Work out the finished part from the listing and answer in its coordinate system (mm). A direction names the side the tool comes from. Round coordinates to 2 decimals unless told otherwise and drop trailing zeros. Write each loop counter-clockwise with the first axis right and the second up, starting at its lowest first coordinate (ties: lowest second). Pieces come first, ordered by that corner, then holes. Notation, with made-up numbers: M 74,-36.5 L 114,-36.5 A4 cw 114,-29.5 Z; hole C -1,62 d1. An arc over 180 degrees is marked long. One line per item, written item: value. Start each with the question number.
Q1. Find section C-C (y = 11). Write down the section's boundary in (x, z) (3 decimals), and give its area (3 significant figures).
Q2. The mould has two halves that part along Y. Classify faces 1 (the flat face through (-0.1, -2.5, 22.86)), 2 (the flat face through (0, -16, 16.51)), 3 (the cylindrical face through (24.85, 14.23, 19.64)): released by +Y, released by -Y, zero draft, split by the parting line, or undercut.
Q3. A tool of negligible diameter and unlimited length cuts with its end or side. For faces 4 (the flat face through (9.8, 11.23, 19.64)), 5 (the cylindrical face through (-18.44, 11.22, 14.94)), 6 (the cylindrical face through (-24.75, 14.41, 19.64)), 7 (the flat face through (-21, 12, 13.335)), 8 (the flat face through (-4.826, -14, 20)), from which of +Z, -Z, +X, -X, +Y, -Y can it reach the whole face along a straight path? Write none if from no direction.
Q4. Find section D-D (y = -14). Write down the section's boundary in (x, z).
Q5. Given pin 1 Ø2.5 at (x, y) = (20, 11) entering from -Z (3 decimals); pin 2 Ø5 at (y, z) = (-15.5, 20.5) entering from -X; pin 3 Ø5 at (y, z) = (-18.5, 19.5) entering from +X, each flat-ended and moving along its own axis, determine where each tip first touches the part or whether it passes through.
Q6. Consider probe 1 along Y at (x, z) = (0, 15); probe 2 along Y at (x, z) = (0, 10); probe 3 along Z at (x, y) = (-10.5, 4). Determine where each line is inside the solid, lowest interval first.
from build123d import *

# Parameters (mm, degrees)
SKETCH1_R           = 6.35
BOSS_EXTRUDE1_DEPTH = 16.51
BOSS_EXTRUDE4_DEPTH = 6.35
SKETCH6_R           = 2.286
BOSS_EXTRUDE5_DEPTH = 3.175
SKETCH7_R           = 2.2225
CUT_EXTRUDE1_DEPTH  = 45.613402568


with BuildPart() as part:
    # Sketch1 → Boss-Extrude1 (new body)
    with BuildSketch(Plane.XY):
        Circle(SKETCH1_R)
    extrude(amount=BOSS_EXTRUDE1_DEPTH)

    # Sketch4 → Boss-Extrude4 (add)
    with BuildSketch(Plane.XY.offset(16.51)):
        with BuildLine():
            Line((-4.826, -4.12701151), (-4.826, -23.8125))
            ThreePointArc((-4.826, -23.8125), (0, -28.6385), (4.826, -23.8125))
            Line((4.826, -23.8125), (4.826, -4.12701151))
            ThreePointArc((4.826, -4.12701151), (5.499261314, -3.175), (5.987096809, -2.115932844))
            Line((5.987096809, -2.115932844), (23.035229928, 7.726811401))
            ThreePointArc((23.035229928, 7.726811401), (24.801668526, 14.31925), (18.209229928, 16.085688599))
            Line((18.209229928, 16.085688599), (1.161096809, 6.242944353))
            ThreePointArc((1.161096809, 6.242944353), (0, 6.35), (-1.161096809, 6.242944353))
            Line((-1.161096809, 6.242944353), (-18.209229928, 16.085688599))
            ThreePointArc((-18.209229928, 16.085688599), (-24.801668526, 14.31925), (-23.035229928, 7.726811401))
            Line((-23.035229928, 7.726811401), (-5.987096809, -2.115932844))
            ThreePointArc((-5.987096809, -2.115932844), (-5.499261314, -3.175), (-4.826, -4.12701151))
        make_face()
    extrude(amount=BOSS_EXTRUDE4_DEPTH)

    # Sketch6 → Boss-Extrude5 (add)
    with BuildSketch(Plane(origin=(0, 0, 16.51), x_dir=(-1, 0, 0), z_dir=(0, 0, -1))):
        with Locations(Location((0, -23.8125, 0), (0, 0, 180))):
            Circle(SKETCH6_R)
        with Locations(Location((-20.622229928, 11.90625, 0), (0, 0, 180))):
            Circle(SKETCH6_R)
        with Locations(Location((20.622229928, 11.90625, 0), (0, 0, 180))):
            Circle(SKETCH6_R)
    extrude(amount=BOSS_EXTRUDE5_DEPTH)

    # Sketch7 → Cut-Extrude1 (cut, through all)
    with BuildSketch(Plane(origin=(0, 0, 0), x_dir=(-1, 0, 0), z_dir=(0, 0, -1))):
        Circle(SKETCH7_R)
    extrude(amount=-CUT_EXTRUDE1_DEPTH, mode=Mode.SUBTRACT)


solid = part.part
The answers:
1. outline: M -25.362,16.51 L -22.721,16.51 L -22.721,13.335 L -18.524,13.335 L -18.524,16.51 L -9.401,16.51 L -9.401,22.86 L -25.362,22.86 Z; M 9.401,16.51 L 18.524,16.51 L 18.524,13.335 L 22.721,13.335 L 22.721,16.51 L 25.362,16.51 L 25.362,22.86 L 9.401,22.86 Z
1. area: 229 mm2
2. face 1: zero draft
2. face 2: undercut
2. face 3: split by the parting line
3. face 4: +Z, -Z, +Y
3. face 5: -Z
3. face 6: +Z, -Z
3. face 7: -Z, +X, -X, +Y, -Y
3. face 8: +Z, -Z, -X, -Y
4. outline: M -4.83,16.51 L 4.83,16.51 L 4.83,22.86 L -4.83,22.86 Z
5. pin 1: z = 13.335
5. pin 2: x = -4.83
5. pin 3: x = 4.83
6. probe 1: -26.1 to -21.53, -6.35 to -2.22, 2.22 to 6.35
6. probe 2: -6.35 to -2.22, 2.22 to 6.35
6. probe 3: 16.51 to 22.86
